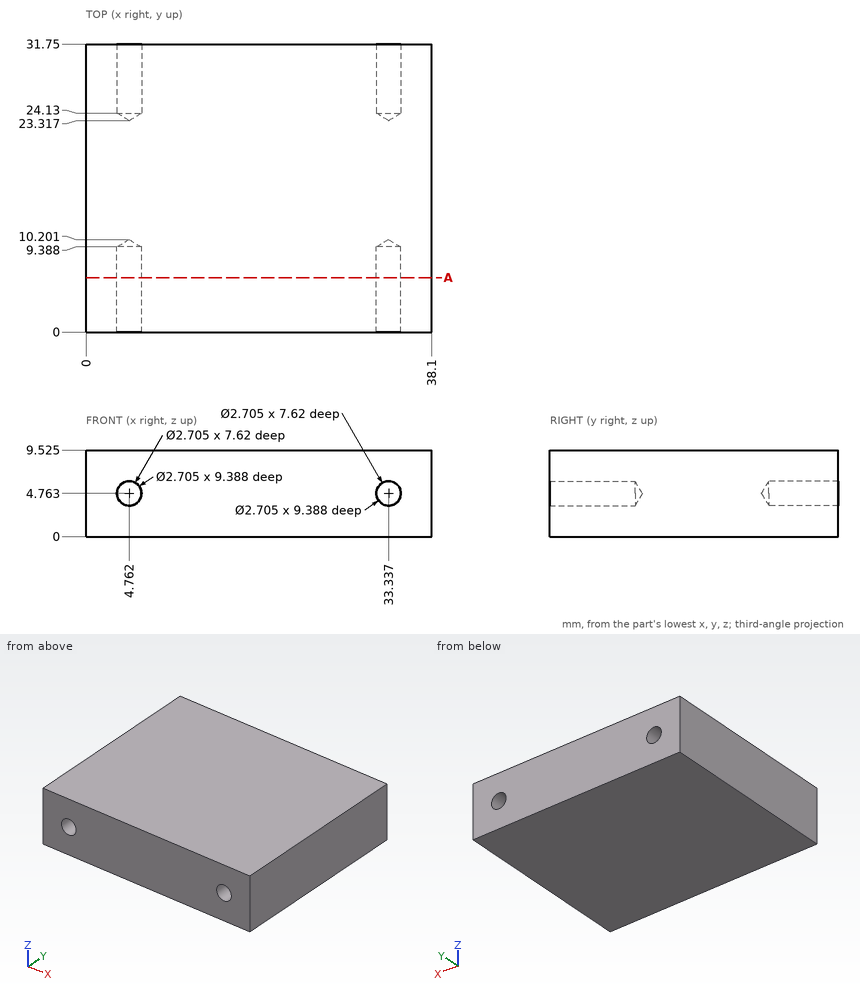
Verification items for this drawing (mm, ordinates from the low corner). Coordinates: 2 decimals unless noted, no trailing zeros. Order: outer loops, then holes, each group sorted by start corner. A loop starts at its lowest first (then second) coordinate and runs counter-clockwise, first axis right, second up. Notation, with made-up numbers: (6, -20) -> (40, -20) arc R19 cw to (40, 9) -> close; hole circle Ø7 at (82, -26.75). An arc over 180 degrees is marked (long way). Put each result on its own line as item: value. Start each with the question number.
1. Cross-section at A-A, the plane y = 6. Record the boundary of the cut face in (x, z) (1 decimal).
2. Material ranges on L1, parallel to X at y = 3.5, z = 3.75 (1 decimal); L2, parallel to X at y = 5.5, z = 5 (1 decimal); L3, parallel to Z at x = 32.5, y = 4 (1 decimal), recorded low to high. Write a range as [from, to].
3. Go/stop test with flat-tipped pins: pin 1 Ø2 at (x, z) = (33.34, 4.76) entering from -Y; pin 2 Ø2.5 at (x, z) = (4.76, 4.76) entering from +Y. Record where each tip stops, or that it passes through.
Computed:
1. outline: (0, 0) -> (38.1, 0) -> (38.1, 9.5) -> (0, 9.5) -> close; hole circle Ø2.7 at (4.8, 4.8); hole circle Ø2.7 at (33.3, 4.8)
2. L1: [0, 3.9], [5.7, 32.4], [34.2, 38.1]
2. L2: [0, 3.4], [6.1, 32], [34.7, 38.1]
2. L3: [0, 3.7], [5.8, 9.5]
3. pin 1: y = 9.6
3. pin 2: y = 24.07
